from build123d import *

# Parameters (mm, degrees)
SKETCH1_W                      = 152.4
SKETCH1_H                      = 50.8
SKETCH1_W_2                    = 142.875
SKETCH1_H_2                    = 41.275
EXTRUDE_THIN1_DEPTH            = 500
M8_CLEARANCE_HOLE1_D           = 9
M8_CLEARANCE_HOLE2_D           = 9
F_12_0_12_DIAMETER_HOLE1_D     = 12
F_12_0_12_DIAMETER_HOLE1_DEPTH = 4.7625
CUT_EXTRUDE1_DEPTH             = 507.41050542
CUT_EXTRUDE1_DEPTH_BACK        = 507.41050542
SKETCH9_R                      = 22.225
M5_CLEARANCE_HOLE1_D           = 5.8
M8_CLEARANCE_HOLE3_D           = 9
M8_CLEARANCE_HOLE3_DEPTH       = 4.7625
F_20_0_20_DIAMETER_HOLE1_D     = 20
F_20_0_20_DIAMETER_HOLE1_DEPTH = 4.7625


with BuildPart() as part:
    # Sketch1 → Extrude-Thin1 (new body)
    with BuildSketch(Plane(origin=(0, 0, 0), x_dir=(1, 0, 0), z_dir=(0, 1, 0))):
        Rectangle(SKETCH1_W, SKETCH1_H)
        Rectangle(SKETCH1_W_2, SKETCH1_H_2, mode=Mode.SUBTRACT)
    extrude(amount=EXTRUDE_THIN1_DEPTH)

    # M8 Clearance Hole1 (through all)
    with Locations(Plane.XY.offset(25.4)):
        with Locations((53.8, 153.666666667), (-56.2, 217), (-16.2, 217), (-56.2, 90.333333333), (53.8, 27)):
            Hole(M8_CLEARANCE_HOLE1_D / 2)

    # M8 Clearance Hole2 (through all)
    with Locations(Plane.XY.offset(25.4)):
        with Locations((-56.2, 367), (-16.2, 247), (-56.2, 247), (-16.2, 367)):
            Hole(M8_CLEARANCE_HOLE2_D / 2)

    # Ø12.0 (12) Diameter Hole1
    with Locations(Plane(origin=(0, 0, -25.4), x_dir=(-1, 0, 0), z_dir=(0, 0, -1))):
        with Locations((36.2, 375.7875), (-13.0125, 425), (36.2, 474.2125)):
            Hole(F_12_0_12_DIAMETER_HOLE1_D / 2, depth=F_12_0_12_DIAMETER_HOLE1_DEPTH)

    # Sketch9 → Cut-Extrude1 (cut, two sides: drawn at the far end of the back side and taken through both)
    with BuildSketch(Plane.XY.offset(-CUT_EXTRUDE1_DEPTH_BACK)):
        with Locations((-36.2, 425)):
            Circle(SKETCH9_R)
    extrude(amount=CUT_EXTRUDE1_DEPTH + CUT_EXTRUDE1_DEPTH_BACK, mode=Mode.SUBTRACT)

    # M5 Clearance Hole1 (through all)
    with Locations(Plane.XY.offset(25.4)):
        with Locations((-44.2, 11), (-8.2, 43), (-8.2, 11), (-44.2, 43)):
            Hole(M5_CLEARANCE_HOLE1_D / 2)

    # M8 Clearance Hole3
    with Locations(Plane(origin=(76.2, 0, 0), x_dir=(0, 0, -1), z_dir=(1, 0, 0))):
        with Locations((-7.9, 50), (-7.9, 10), (7.1, 30)):
            Hole(M8_CLEARANCE_HOLE3_D / 2, depth=M8_CLEARANCE_HOLE3_DEPTH)

    # Ø20.0 (20) Diameter Hole1
    with Locations(Plane.ZY.offset(76.2)):
        with Locations((0.4, 40)):
            Hole(F_20_0_20_DIAMETER_HOLE1_D / 2, depth=F_20_0_20_DIAMETER_HOLE1_DEPTH)


solid = part.part
Geometry check sheet. Reference: the model listing, model coordinates, mm. A direction names the side the tool comes from. Coordinates: 2 decimals unless noted, no trailing zeros. Order: outer loops, then holes, each group sorted by start corner. A loop starts at its lowest first (then second) coordinate and runs counter-clockwise, first axis right, second up. Notation, with made-up numbers: (26.5, -35.5) - (70.5, -35.5) arc R16 cw to (70.5, -14.5) - close; hole circle Ø6 at (75, -21.75). An arc over 180 degrees is marked (long way). Answer in a Markdown table with one row per item. Add a question column.
1) Gauge pin test, flat ends, axial feed: P1, Ø3.5, axis at x = -8.2, y = 43, coming from the +Z side; P2, Ø7.5, axis at x = -44.2, y = 43, coming from the +Z side; P3, Ø7, axis at y = 50, z = 7.9, coming from the +X side. Record the tip position at first contact, or that the pin passes through.
2) Cross-section at A-A, the plane x = 63. Record the cut outline in (y, z), then the cut area to 3 significant figures.
3) Release check for a two-part mould opening along Y. For faces 5 (the cylindrical face through (-15.22, 212.61, 22.99)), 6 (the flat face through (-6, 0, -21)), 7 (the flat face through (76.2, 246, 0)) record: +Y half, -Y half, draft (parallel to the pull), parting line (faces both ways), or undercut.
4) Cross-section at B-B, the plane y = 335.5. Record the cut outline in (x, z).
5) Material ranges on line 1 along X through (y, z) = (425, -24) (1 decimal); line 2 along X through (y, z) = (413.5, 14.5); line 3 along Z through (x, y) = (-45, 337), recorded low to high. Write a range as [from, to].
6) Set-up check for faces 1 (the cylindrical face through (49.508, 28.352, -23.052)), 2 (the cylindrical face through (-73.79, 30.24, 2.57)), 3 (the flat face through (-1, 246, -20.638)), 4 (the cylindrical face through (73.785, 11.352, 12.192)): record each of +Z, -Z, +X, -X, +Y, -Y from which the full face is reachable in a straight line by a thin tool's end or side.
Check result:
| question | item | result |
|---|---|---|
| 1 | P1 | passes through |
| 1 | P2 | stops at z = 25.4 |
| 1 | P3 | stops at x = -71.44 |
| 2 | outline | (0, -25.4) - (500, -25.4) - (500, -20.64) - (0, -20.64) - close; (0, 20.64) - (500, 20.64) - (500, 25.4) - (0, 25.4) - close |
| 2 | area | 4,760 mm² |
| 3 | face 5 | undercut |
| 3 | face 6 | -Y half |
| 3 | face 7 | draft |
| 4 | outline | (-76.2, -25.4) - (76.2, -25.4) - (76.2, 25.4) - (-76.2, 25.4) - close; hole (-71.44, -20.64) - (71.44, -20.64) - (71.44, 20.64) - (-71.44, 20.64) - close |
| 5 | line 1 | x = [-76.2, -58.4], [-14, 7], [19, 76.2] |
| 5 | line 2 | x = [-76.2, -71.44], [71.44, 76.2] |
| 5 | line 3 | z = [-25.4, -20.64], [20.64, 25.4] |
| 6 | face 1 | +Z, -Z |
| 6 | face 2 | -X |
| 6 | face 3 | +Y, -Y |
| 6 | face 4 | +X |
